Could you check a few things on this model? Use its own coordinates, in mm. A direction names the side the tool comes from. Coordinates: 2 decimals unless noted, no trailing zeros. Order: outer loops, then holes, each group sorted by start corner. A loop starts at its lowest first (then second) coordinate and runs counter-clockwise, first axis right, second up. Notation, with made-up numbers: (-10.75, 25) - (2.25, 25) arc R8 cw to (2.25, 30) - close; hole circle Ø6 at (50, -37.5). An arc over 180 degrees is marked (long way). Answer as CSV lines item,"result". Start each with the question number.
1. I want a section at C-C, the plane y = 98. List the corners of the cut face in (x, z) for me.
2. I want a section at D-D, the plane y = 65.5. List the corners of the cut face in (x, z) for me (3 decimals).
3. I need wall thicknesses on probe 1 along Z at (x, y) = (-1.5, 19.5) (3 decimals); probe 2 along Y at (x, z) = (1.25, 3); probe 3 along Z at (x, y) = (-1, 94.5). Which ranges of each line are inside material? Lowest first, please.
4. I want a section at B-B, the plane z = 0. List the corners of the cut face in (x, y) for me (3 decimals).
5. For faces 1 (the face through (-2, 90, -2)), 2 (the face through (0, 100, 1.8)), 3 (the face through (2.64, 9.86, 0.03)), 4 (the face through (0, 20, -2)), which set-ups out of +Z, -Z, +X, -X, +Y, -Y let a thin tool reach every point of the face, with its end or its side?
6. I want a section at A-A, the plane x = 0. List the corners of the cut face in (y, z) for me (3 decimals).
7. For pin 1 (4 mm diameter, centred on x = -3, z = -2.5, fed in from +Y); pin 2 (1.1 mm diameter, centred on x = 0, y = 8.5, fed in from -Z) (3 decimals); pin 3 (4 mm diameter, centred on y = 12.5, z = -1.5, fed in from -X); pin 4 (1.2 mm diameter, centred on x = 0, y = 102.5, fed in from +Z), each with a flat end and sliding along its axis, tell me the tip position at first contact or that it passes through.
from build123d import *

# Parameters (mm, degrees)
BOSS_EXTRUDE1_DEPTH = 20
SKETCH2_R           = 4.075
BOSS_EXTRUDE2_DEPTH = 70
BOSS_EXTRUDE3_DEPTH = 20


with BuildPart() as part:
    # Sketch1 → Boss-Extrude1 (new body)
    with BuildSketch(Plane(origin=(0, 0, 0), x_dir=(1, 0, 0), z_dir=(0, 1, 0))):
        with BuildLine():
            Line((1.907609761, 1.825), (-1.907609761, 1.825))
            ThreePointArc((-1.907609761, 1.825), (-2.64, 0), (-1.907609761, -1.825))
            Line((-1.907609761, -1.825), (1.907609761, -1.825))
            ThreePointArc((1.907609761, -1.825), (2.64, 0), (1.907609761, 1.825))
        make_face()
    extrude(amount=BOSS_EXTRUDE1_DEPTH)

    # Sketch2 → Boss-Extrude2 (add)
    with BuildSketch(Plane(origin=(0, 20, 0), x_dir=(1, 0, 0), z_dir=(0, 1, 0))):
        with Locations(Location((0, 0, 0), (0, 0, 270))):
            Circle(SKETCH2_R)
    extrude(amount=BOSS_EXTRUDE2_DEPTH)

    # Sketch3 → Boss-Extrude3 (add)
    with BuildSketch(Plane(origin=(0, 90, 0), x_dir=(1, 0, 0), z_dir=(0, 1, 0))):
        with BuildLine():
            Line((1.897366596, 1.85), (-1.897366596, 1.85))
            ThreePointArc((-1.897366596, 1.85), (-2.649775646, 0.034482248), (-1.944865034, -1.8))
            Line((-1.944865034, -1.8), (1.944865034, -1.8))
            ThreePointArc((1.944865034, -1.8), (2.649775646, 0.034482248), (1.897366596, 1.85))
        make_face()
    extrude(amount=BOSS_EXTRUDE3_DEPTH)


solid = part.part
Solved:
1,outline,"(-1.94, 1.8) arc R2.65 ccw to (-1.9, -1.85) - (1.9, -1.85) arc R2.65 ccw to (1.94, 1.8) - close"
2,outline,"circle Ø8.15 at (0, 0)"
3,probe 1,"z = -1.825 to 1.825"
3,probe 2,"y = 20 to 90"
3,probe 3,"z = -1.85 to 1.8"
4,outline,"(-4.075, 20) - (-2.64, 20) - (-2.64, 0) - (2.64, 0) - (2.64, 20) - (4.075, 20) - (4.075, 90) - (2.65, 90) - (2.65, 110) - (-2.65, 110) - (-2.65, 90) - (-4.075, 90) - close"
5,face 1,"+Y"
5,face 2,"+Z, +X, -X, +Y"
5,face 3,"+X, -Y"
5,face 4,"-Y"
6,outline,"(0, -1.825) - (20, -1.825) - (20, -4.075) - (90, -4.075) - (90, -1.85) - (110, -1.85) - (110, 1.8) - (90, 1.8) - (90, 4.075) - (20, 4.075) - (20, 1.825) - (0, 1.825) - close"
7,pin 1,"stops at y = 110"
7,pin 2,"stops at z = -1.825"
7,pin 3,"stops at x = -2.64"
7,pin 4,"stops at z = 1.8"
